For this review, take the finished solid that the model builds, in its own axes (mm). Face numbers are marked on the shaded views. A direction names the side the tool comes from. Give positions to 0.01 mm unless a question says otherwise; leave off trailing zeros. Write each loop counter-clockwise with the first axis right and the second up, starting at its lowest first coordinate (ties: lowest second). Pieces come first, ordered by that corner, then holes. Notation, with made-up numbers: (66, 13) -> (89, 13) arc R11 ccw to (89, 21) -> close; hole circle Ø1 at (87, 57.25). An arc over 180 degrees is marked (long way). Answer as CSV lines item,"result".
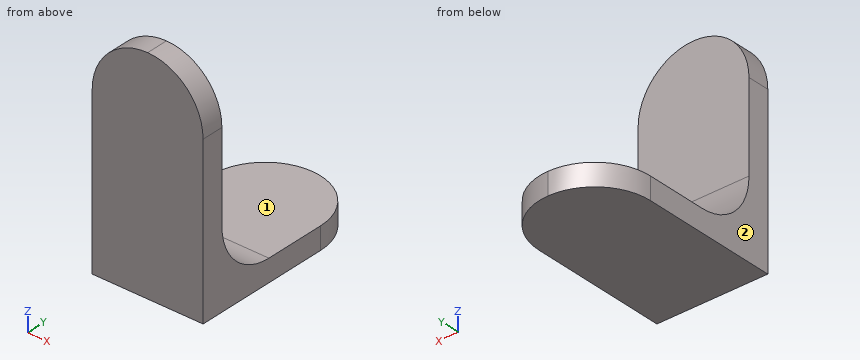
```python
from build123d import *

# Parameters (mm, degrees)
F0_W     = 4
F0_H     = 4
F0_W_2   = 31
F0_H_2   = 36
F1_DEPTH = 10
F2_R     = 9.99999


# Not quite as in the source:
# - a fillet or chamfer is up to 0.001 mm smaller than in the source, because OpenCascade refuses the exact size


with BuildPart() as f1:
    # F0 (on Right) → F1 (new body, symmetric)
    with BuildSketch(Plane.YZ):
        with Locations((2, 2)):
            Rectangle(F0_W, F0_H)
        with Locations((19.5, 2)):
            Rectangle(F0_W_2, F0_H)
        with Locations((2, 22)):
            Rectangle(F0_W, F0_H_2)
    extrude(amount=F1_DEPTH, both=True)

    # F2 (radius 10 in the source; OpenCascade refuses exactly that, so slightly less here)
    f2_edges = [f1.edges().sort_by_distance(p)[0] for p in [
        (0, 4, 4),
        (10, 35, 2),
        (-10, 35, 2),
        (10, 2, 40),
        (-10, 2, 40),
    ]]
    fillet(f2_edges, radius=F2_R)


solid = f1.part
```
Q1. Add section B-B (z = 15). Write out the cut boundary in (x, y), plus the area to 3 significant figures.
Answer block:
outline,"(-10, 0) -> (10, 0) -> (10, 4) -> (-10, 4) -> close"
area,"80.0 mm2"
Q2. Add section A-A (x = -4.75). Write out the cut boundary in (y, z), plus the area to 3 significant figures.
Answer block:
outline,"(0, 0) -> (33.8, 0) -> (33.8, 4) -> (14, 4) arc R10 cw to (4, 14) -> (4, 38.8) -> (0, 38.8) -> close"
area,"296 mm2"
Q3. Add section C-C (y = 33). Write out the cut boundary in (x, z).
Answer block:
outline,"(-6, 0) -> (6, 0) -> (6, 4) -> (-6, 4) -> close"
Q4. Add section D-D (x = 2). Write out the cut boundary in (y, z).
Answer block:
outline,"(0, 0) -> (34.8, 0) -> (34.8, 4) -> (14, 4) arc R10 cw to (4, 14) -> (4, 39.8) -> (0, 39.8) -> close"
Q5. To check wall thickness, follow probe 1 along Y at (x, z) = (8, 33.5); probe 2 along Z at (x, y) = (9, 7). State the ranges of each line that lie inside material, in increasing order. Write a range as [from, to].
Answer block:
probe 1,"y = [0, 4]"
probe 2,"z = [0, 6.86]"
Q6. For the marked faces 1 and 2, list the 3-axis set-ups (+Z, -Z, +X, -X, +Y, -Y) from which the entire face can be reached by the end or side of a thin tool; tool diameter is ignored.
Answer block:
face 1,"+Z, +X, -X, +Y"
face 2,"+Z, -Z, -X, +Y, -Y"
Q7. Clearance check with flat-ended pins moving along their axes: pin 1 (4 mm diameter, centred on x = 0, y = 20, fed in from +Z); pin 2 (4 mm diameter, centred on x = -5, y = 7, fed in from +Z). State where each tip first meets the part, or that it passes through.
Answer block:
pin 1,"stops at z = 4"
pin 2,"stops at z = 9.64"
